Design review of the part built by this model. Coordinates are the model's own, in mm. A direction names the side the tool comes from. Coordinates: 2 decimals unless noted, no trailing zeros. Loops run counter-clockwise (first coordinate to the right, second up) from the corner with the lowest first, then second, coordinate; pieces in that order, holes last.
Q1. Add section A-A on x = 0. Give the boundary of the cut face in (y, z).
Q2. Wall thickness on probe 1 along X at (y, z) = (4.25, 0); probe 2 along Y at (x, z) = (-16, -2); probe 3 along X at (y, z) = (4.5, 14): over which ranges is each line inside the solid? List them lowest first.
Q3. For P1, Ø11, axis at x = -12, z = 0, coming from the +Y side; P2, Ø2, axis at x = 4.5, y = 5.5, coming from the -Z side; P3, Ø13, axis at x = 0, z = 0, coming from the +Y side; P4, Ø5.5, axis at x = 12, z = 0, coming from the -Y side, all flat-tipped, find the tip position at first contact; note any pin that passes through.
Q4. Add section B-B on z = 0. Give the boundary of the cut face in (x, y).
Q5. Machinability: for faces 4 (the face through (0, 0, 5)), 5 (the face through (4, 7, 4)), which of the approach directions +Z, -Z, +X, -X, +Y, -Y give a long, thin tool a straight path to every point of the face, cutting with its end or side? Answer none if there is none.
Q6. Draft analysis for pull direction X (two halves, no side actions). For faces 1 (the face through (-12, 9, -14)), 2 (the face through (0.154, 3.451, 8.503)), 3 (the face through (7.21, 4.45, 22.89)), state which applies: released by +X, released by -X, zero draft, split by the parting line, or undercut.
Q7. Add section C-C on y = 5.5. Give the boundary of the cut face in (x, z), and give its area (3 significant figures).
```python
from build123d import *

# Parameters (mm, degrees)
SKETCH2_R           = 24
SKETCH2_R_2         = 18
BOSS_EXTRUDE2_DEPTH = 9
SKETCH2_3_R         = 18
SKETCH2_3_R_2       = 16
SKETCH2_3_R_3       = 3.5
SKETCH2_3_R_4       = 4
BOSS_EXTRUDE3_DEPTH = 7
CHAMFER1_SIZE       = 1
CHAMFER3_SIZE       = 1


with BuildPart() as part:
    # Sketch2 → Boss-Extrude2 (new body)
    with BuildSketch(Plane(origin=(0, 0, 0), x_dir=(1, 0, 0), z_dir=(0, 1, 0))):
        with Locations(Location((0, 0, 0), (0, 0, 270))):
            Circle(SKETCH2_R)
        with Locations(Location((0, 0, 0), (0, 0, 270))):
            Circle(SKETCH2_R_2, mode=Mode.SUBTRACT)
    extrude(amount=BOSS_EXTRUDE2_DEPTH)

    # Sketch2_3 → Boss-Extrude3 (add)
    # profile 1 of 2: a face of its own
    with BuildSketch(Plane(origin=(0, 0, 0), x_dir=(1, 0, 0), z_dir=(0, 1, 0))):
        with Locations(Location((0, 0, 0), (0, 0, 270))):
            Circle(SKETCH2_3_R)
        Circle(SKETCH2_3_R_2, mode=Mode.SUBTRACT)
    # profile 2 of 2: a face of its own
    with BuildSketch(Plane(origin=(0, 0, 0), x_dir=(1, 0, 0), z_dir=(0, 1, 0))):
        Circle(SKETCH2_3_R_2)
        with Locations(Location((-12, 0, 0), (0, 0, 270))):
            Circle(SKETCH2_3_R_3, mode=Mode.SUBTRACT)
        with Locations(Location((0, -12, 0), (0, 0, 270))):
            Circle(SKETCH2_3_R_3, mode=Mode.SUBTRACT)
        with Locations(Location((12, 0, 0), (0, 0, 270))):
            Circle(SKETCH2_3_R_3, mode=Mode.SUBTRACT)
        with Locations(Location((0, 12, 0), (0, 0, 270))):
            Circle(SKETCH2_3_R_3, mode=Mode.SUBTRACT)
        with Locations(Location((0, 0, 0), (0, 0, 270))):
            Circle(SKETCH2_3_R_4, mode=Mode.SUBTRACT)
    extrude(amount=BOSS_EXTRUDE3_DEPTH)

    # Chamfer1
    chamfer1_edges = [part.edges().sort_by_distance(p)[0] for p in [
        (0, 9, -24),
        (0, 0, -24),
    ]]
    chamfer(chamfer1_edges, length=CHAMFER1_SIZE)

    # Chamfer3
    chamfer3_edges = [part.edges().sort_by_distance(p)[0] for p in [
        (0, 7, -18),
    ]]
    chamfer(chamfer3_edges, length=CHAMFER3_SIZE)


solid = part.part
```
Entries:
1. outline: (0, -23) - (1, -24) - (8, -24) - (9, -23) - (9, -18) - (8, -18) - (7, -17) - (7, -15.5) - (0, -15.5) - close; (0, -8.5) - (7, -8.5) - (7, -4) - (0, -4) - close; (0, 4) - (7, 4) - (7, 8.5) - (0, 8.5) - close; (0, 15.5) - (7, 15.5) - (7, 17) - (8, 18) - (9, 18) - (9, 23) - (8, 24) - (1, 24) - (0, 23) - close
2. probe 1: x = -24 to -15.5, -8.5 to -4, 4 to 8.5, 15.5 to 24
2. probe 2: y = 0 to 7
2. probe 3: x = -19.49 to -2.87, 2.87 to 19.49
3. P1: stops at y = 7.5
3. P2: stops at z = -23.74
3. P3: stops at y = 7
3. P4: passes through
4. outline: (-24, 1) - (-23, 0) - (-15.5, 0) - (-15.5, 7) - (-17, 7) - (-18, 8) - (-18, 9) - (-23, 9) - (-24, 8) - close; (-8.5, 0) - (-4, 0) - (-4, 7) - (-8.5, 7) - close; (4, 0) - (8.5, 0) - (8.5, 7) - (4, 7) - close; (15.5, 0) - (23, 0) - (24, 1) - (24, 8) - (23, 9) - (18, 9) - (18, 8) - (17, 7) - (15.5, 7) - close
5. face 4: +Z, -Z, +X, -X, -Y
5. face 5: +Y
6. face 1: zero draft
6. face 2: undercut
6. face 3: split by the parting line
7. outline: circle Ø48 at (0, 0); hole circle Ø7 at (-12, 0); hole circle Ø8 at (0, 0); hole circle Ø7 at (0, -12); hole circle Ø7 at (0, 12); hole circle Ø7 at (12, 0)
7. area: 1,610 mm2
